Geometry check sheet. Reference: the model listing, model coordinates, mm. A direction names the side the tool comes from. Give positions to 0.01 mm unless a question says otherwise; leave off trailing zeros. Write each loop counter-clockwise with the first axis right and the second up, starting at its lowest first coordinate (ties: lowest second). Pieces come first, ordered by that corner, then holes. Notation, with made-up numbers: (82.25, 7) -> (125.25, 7) arc R5 ccw to (125.25, 16) -> close; hole circle Ø9 at (66.5, 73.5). An arc over 180 degrees is marked (long way). One line per item, written item: value.
from build123d import *

# Parameters (mm, degrees)
SKETCH1_W           = 404
SKETCH1_H           = 160
BOSS_EXTRUDE1_DEPTH = 3


with BuildPart() as part:
    # Sketch1 → Boss-Extrude1 (new body)
    with BuildSketch(Plane.XY.offset(152)):
        with Locations((134.5, -85.941341737)):
            Rectangle(SKETCH1_W, SKETCH1_H)
        with BuildLine():
            Line((-47.5, -138.822974494), (-47.5, -33.059708979))
            ThreePointArc((-47.5, -33.059708979), (-45.373921063, -28.968183869), (-40.80376891, -28.356220902))
            Line((-40.80376891, -28.356220902), (105.831987613, -81.23785366))
            ThreePointArc((105.831987613, -81.23785366), (109.135756522, -85.941341737), (105.831987613, -90.644829813))
            Line((105.831987613, -90.644829813), (-40.80376891, -143.526462571))
            ThreePointArc((-40.80376891, -143.526462571), (-45.373921063, -142.914499604), (-47.5, -138.822974494))
        make_face(mode=Mode.SUBTRACT)
        with BuildLine():
            Line((228.942684704, -25.941341737), (40.057315296, -25.941341737))
            ThreePointArc((40.057315296, -25.941341737), (35.132001073, -30.080365658), (38.361084206, -35.644829813))
            Line((38.361084206, -35.644829813), (132.80376891, -69.703939867))
            ThreePointArc((132.80376891, -69.703939867), (134.5, -70.00045179), (136.19623109, -69.703939867))
            Line((136.19623109, -69.703939867), (230.638915794, -35.644829813))
            ThreePointArc((230.638915794, -35.644829813), (233.867998927, -30.080365658), (228.942684704, -25.941341737))
        make_face(mode=Mode.SUBTRACT)
        with BuildLine():
            Line((309.80376891, -28.356220902), (163.168012387, -81.23785366))
            ThreePointArc((163.168012387, -81.23785366), (159.864243478, -85.941341737), (163.168012387, -90.644829813))
            Line((163.168012387, -90.644829813), (309.80376891, -143.526462571))
            ThreePointArc((309.80376891, -143.526462571), (314.373921063, -142.914499604), (316.5, -138.822974494))
            Line((316.5, -138.822974494), (316.5, -33.059708979))
            ThreePointArc((316.5, -33.059708979), (314.373921063, -28.968183869), (309.80376891, -28.356220902))
        make_face(mode=Mode.SUBTRACT)
        with BuildLine():
            Line((38.361084206, -136.23785366), (132.80376891, -102.178743606))
            ThreePointArc((132.80376891, -102.178743606), (134.5, -101.882231683), (136.19623109, -102.178743606))
            Line((136.19623109, -102.178743606), (230.638915794, -136.23785366))
            ThreePointArc((230.638915794, -136.23785366), (233.867998927, -141.802317815), (228.942684704, -145.941341737))
            Line((228.942684704, -145.941341737), (40.057315296, -145.941341737))
            ThreePointArc((40.057315296, -145.941341737), (35.132001073, -141.802317815), (38.361084206, -136.23785366))
        make_face(mode=Mode.SUBTRACT)
    extrude(amount=BOSS_EXTRUDE1_DEPTH)


solid = part.part
1) Scan lines: probe 1 along Y at (x, z) = (203, 153.15); probe 2 along Y at (x, z) = (212.5, 154.8); probe 3 along Y at (x, z) = (131.5, 154.55). Record each from-to range of solid material in increasing order.
Verdict:
probe 1: -165.94 to -145.94, -126.27 to -105.01, -66.87 to -45.61, -25.94 to -5.94
probe 2: -165.94 to -145.94, -129.7 to -108.44, -63.45 to -42.19, -25.94 to -5.94
probe 3: -165.94 to -145.94, -102.65 to -69.23, -25.94 to -5.94
2) Sectioned sample at C-C on x = 101.5. Record the cut outline in (y, z), plus the area to 3 significant figures.
Verdict:
outline: (-165.94, 152) -> (-145.94, 152) -> (-145.94, 155) -> (-165.94, 155) -> close; (-113.47, 152) -> (-92.21, 152) -> (-92.21, 155) -> (-113.47, 155) -> close; (-79.68, 152) -> (-58.41, 152) -> (-58.41, 155) -> (-79.68, 155) -> close; (-25.94, 152) -> (-5.94, 152) -> (-5.94, 155) -> (-25.94, 155) -> close
area: 248 mm^2
3) Sectioned sample at D-D on y = -44. Record the cut outline in (x, z).
Verdict:
outline: (-67.5, 152) -> (-47.5, 152) -> (-47.5, 155) -> (-67.5, 155) -> close; (2.57, 152) -> (61.53, 152) -> (61.53, 155) -> (2.57, 155) -> close; (207.47, 152) -> (266.43, 152) -> (266.43, 155) -> (207.47, 155) -> close; (316.5, 152) -> (336.5, 152) -> (336.5, 155) -> (316.5, 155) -> close
4) Mould release check, pull along Y, two halves, no side actions. Record for faces 1 (the flat face through (87, -103, 155)), 2 (the flat face through (84.921, -52.436, 153.479)): released by +Y, released by -Y, zero draft, split by the parting line, or undercut.
Verdict:
face 1: zero draft
face 2: undercut
5) Sectioned sample at B-B on z = 153.7. Record the cut outline in (x, y).
Verdict:
outline: (-67.5, -165.94) -> (336.5, -165.94) -> (336.5, -5.94) -> (-67.5, -5.94) -> close; hole (-47.5, -138.82) arc R5 ccw to (-40.8, -143.53) -> (105.83, -90.64) arc R5 ccw to (105.83, -81.24) -> (-40.8, -28.36) arc R5 ccw to (-47.5, -33.06) -> close; hole (38.36, -136.24) arc R5 ccw to (40.06, -145.94) -> (228.94, -145.94) arc R5 ccw to (230.64, -136.24) -> (136.2, -102.18) arc R5 ccw to (132.8, -102.18) -> close; hole (38.36, -35.64) -> (132.8, -69.7) arc R5 ccw to (136.2, -69.7) -> (230.64, -35.64) arc R5 ccw to (228.94, -25.94) -> (40.06, -25.94) arc R5 ccw to start; hole (163.17, -90.64) -> (309.8, -143.53) arc R5 ccw to (316.5, -138.82) -> (316.5, -33.06) arc R5 ccw to (309.8, -28.36) -> (163.17, -81.24) arc R5 ccw to start
6) Tool access check on faces 3 (the flat face through (31.488, -54.427, 153.479)), 4 (the flat face through (87, -103, 152)). Record the directions out of +Z, -Z, +X, -X, +Y, -Y that give a thin tool (end or side, any length) a straight path to the whole face; none if there is none.
Verdict:
face 3: +Z, -Z
face 4: -Z, +X, -X, +Y, -Y
7) Sectioned sample at A-A on x = 155. Record the cut outline in (y, z), plus the area to 3 significant figures.
Verdict:
outline: (-165.94, 152) -> (-145.94, 152) -> (-145.94, 155) -> (-165.94, 155) -> close; (-108.96, 152) -> (-62.92, 152) -> (-62.92, 155) -> (-108.96, 155) -> close; (-25.94, 152) -> (-5.94, 152) -> (-5.94, 155) -> (-25.94, 155) -> close
area: 258 mm^2
